```python
from build123d import *

# Parameters (mm, degrees)
SKETCH1_W                  = 8
SKETCH1_H                  = 17
CONNECTOR_BODY_DEPTH       = 8
SKETCH4_W                  = 4
SKETCH4_H                  = 16
CLAMP_DEPTH                = 2
CONNECTOR_PATTERN_COUNT    = 2
CONNECTOR_PATTERN_PITCH    = 5
SKETCH5_W                  = 8
SKETCH5_H                  = 12.5
SINGLE_BODY_DEPTH          = 8
SKETCH6_W                  = 1.5
SKETCH6_H                  = 2.500390225
CHAINING_NOBS_DEPTH        = 1
SKETCH7_W                  = 1.10359402
SKETCH7_H                  = 1.518729337
SKETCH7_H_2                = 1.556223895
CHAINING_NOBS_CUTOUT_DEPTH = 2.5
SKETCH8_W                  = 4
SKETCH8_H                  = 12.5
SINGLE_BODY_CLAMP_DEPTH    = 2


with BuildPart() as part:
    # Sketch1 → connector_body (new body)
    with BuildSketch(Plane(origin=(0, 0, 0), x_dir=(1, 0, 0), z_dir=(0, 1, 0))):
        with Locations((4, 8.5)):
            Rectangle(SKETCH1_W, SKETCH1_H)
    connector_body = extrude(amount=CONNECTOR_BODY_DEPTH)

    # Sketch3 → cable_hole (revolve, cut)
    with BuildSketch(Plane(origin=(4, 4, 0), x_dir=(0, -1, 0), z_dir=(1, 0, 0))):
        Polygon((0, 0), (0, 10.600860619), (1, 10), (1, 0.025), (1.025, 0), align=None)
    cable_hole = revolve(axis=Axis((4, 4, 6.35), (0, 0, -1)), mode=Mode.SUBTRACT)

    # Sketch4 → clamp (add)
    with BuildSketch(Plane(origin=(0, 8, 0), x_dir=(1, 0, 0), z_dir=(0, 1, 0))):
        with Locations((4, 6)):
            Rectangle(SKETCH4_W, SKETCH4_H)
    clamp = extrude(amount=CLAMP_DEPTH)

    # connector_pattern: connector_body, cable_hole, clamp ×2
    with Locations(*[(i * CONNECTOR_PATTERN_PITCH, 0, 0) for i in range(1, CONNECTOR_PATTERN_COUNT)]):
        add(connector_body)
        add(cable_hole, mode=Mode.SUBTRACT)
        add(clamp)

    # Sketch5 → single_body (add)
    with BuildSketch(Plane(origin=(0, 8, 0), x_dir=(1, 0, 0), z_dir=(0, 1, 0))):
        with Locations((6.5, 23.25)):
            Rectangle(SKETCH5_W, SKETCH5_H)
    extrude(amount=-SINGLE_BODY_DEPTH)

    # Sketch6 → chaining_nobs (add)
    with BuildSketch(Plane.ZY):
        with Locations((-11.25, 1.250195113)):
            Rectangle(SKETCH6_W, SKETCH6_H)
        with Locations((-4.75, 1.250195113)):
            Rectangle(SKETCH6_W, SKETCH6_H)
    extrude(amount=CHAINING_NOBS_DEPTH)

    # Sketch7 → chaining_nobs_cutout (cut)
    with BuildSketch(Plane.XZ):
        with Locations((12.44820299, -4.740635332)):
            Rectangle(SKETCH7_W, SKETCH7_H)
        with Locations((12.44820299, -11.278111948)):
            Rectangle(SKETCH7_W, SKETCH7_H_2)
    extrude(amount=-CHAINING_NOBS_CUTOUT_DEPTH, mode=Mode.SUBTRACT)

    # Sketch8 → single_body_clamp (add)
    with BuildSketch(Plane(origin=(0, 8, 0), x_dir=(1, 0, 0), z_dir=(0, 1, 0))):
        with Locations((6.5, 25.25)):
            Rectangle(SKETCH8_W, SKETCH8_H)
    extrude(amount=SINGLE_BODY_CLAMP_DEPTH)


solid = part.part
```
Work out the finished part from the listing and answer in its coordinate system (mm). A direction names the side the tool comes from. Give positions to 0.01 mm unless a question says otherwise; leave off trailing zeros. Order: outer loops, then holes, each group sorted by start corner. A loop starts at its lowest first (then second) coordinate and runs counter-clockwise, first axis right, second up.
1. Section C-C, the plane x = 6.5 is taken. Determine the outline of the cut face in (y, z).
Result sheet:
outline: (0, -29.5) - (8, -29.5) - (8, -31.5) - (10, -31.5) - (10, -19) - (8, -19) - (8, 0) - (0, 0) - close
2. Each of these flat-tipped pins is pushed along its axis until it touches: P1, Ø1, axis at x = 6, y = 3, coming from the -Z side; P2, Ø1, axis at y = 9, z = -9.5, coming from the -X side; P3, Ø2.5, axis at y = 3.5, z = -23.5, coming from the -X side; P4, Ø1.5, axis at x = 6.5, z = -4, coming from the +Y side. Where does it stop, or does it pass through?
Result sheet:
P1: stops at z = -29.5
P2: stops at x = 2
P3: stops at x = 2.5
P4: stops at y = 10
3. Section D-D, the plane x = 1 is taken. Determine the outline of the cut face in (y, z), and give its area (3 significant figures).
Result sheet:
outline: (0, -17) - (8, -17) - (8, 0) - (0, 0) - close
area: 136 mm2
4. Section B-B, the plane z = -28.5 is taken. Determine the outline of the cut face in (x, y).
Result sheet:
outline: (2.5, 0) - (10.5, 0) - (10.5, 8) - (8.5, 8) - (8.5, 10) - (4.5, 10) - (4.5, 8) - (2.5, 8) - close
5. Section A-A, the plane y = 1.25 is taken. Determine the outline of the cut face in (x, z).
Result sheet:
outline: (-1, -12) - (0, -12) - (0, -17) - (2.5, -17) - (2.5, -29.5) - (10.5, -29.5) - (10.5, -17) - (13, -17) - (13, -12.06) - (11.9, -12.06) - (11.9, -10.5) - (13, -10.5) - (13, -5.5) - (11.9, -5.5) - (11.9, -3.98) - (13, -3.98) - (13, 0) - (0, 0) - (0, -4) - (-1, -4) - (-1, -5.5) - (0, -5.5) - (0, -10.5) - (-1, -10.5) - close
6. Straight lines are drawn through the part: L1, parallel to X at y = 4, z = -4.5; L2, parallel to Y at x = 4, z = -8.5; L3, parallel to X at y = 8.5, z = -5.5. For each, find the intervals that lie inside material, in ascending order.
Result sheet:
L1: x = 0 to 3, 5 to 8, 10 to 13
L2: y = 0 to 3, 5 to 10
L3: x = 2 to 6, 7 to 11
7. The mould has two halves that part along Z. Classify faces 1 (the flat face through (9, 10, -6)), 2 (the flat face through (9, 9, 2)), 3 (the flat face through (12.4, 1.2, -5.5)): released by +Z, released by -Z, zero draft, split by the parting line, or undercut.
Result sheet:
face 1: zero draft
face 2: released by +Z
face 3: undercut
8. For faces 4 (the flat face through (12.4, 2.5, -11.3)), 5 (the flat face through (-0.5, 2.5, -4.8)), 6 (the flat face through (9, 9, -14)), determine the directions among +Z, -Z, +X, -X, +Y, -Y from which every point of the face is accessible in a straight line to the end or side of a thin tool.
Result sheet:
face 4: +X, -Y
face 5: +Z, -Z, -X, +Y
face 6: +X, -X, +Y
